```python
from build123d import *

# Parameters (mm, degrees)
SKETCH1_W           = 12.7
SKETCH1_H           = 12.7
BOSS_EXTRUDE1_DEPTH = 6.35
SKETCH2_W           = 1.016
SKETCH2_H           = 3.5052
BOSS_EXTRUDE2_DEPTH = 6.35
FILLET1_R           = 0.635
FILLET2_R           = 0.254


with BuildPart() as part:
    # Sketch1 → Boss-Extrude1 (new body)
    with BuildSketch(Plane(origin=(0, 0, 0), x_dir=(1, 0, 0), z_dir=(0, 1, 0))):
        Rectangle(SKETCH1_W, SKETCH1_H)
    extrude(amount=BOSS_EXTRUDE1_DEPTH)

    # Sketch2 → Boss-Extrude2 (add)
    with BuildSketch(Plane.XY.offset(6.35)):
        with Locations((-2.624666667, 3.175)):
            Rectangle(SKETCH2_W, SKETCH2_H)
        with Locations((2.624666667, 3.175)):
            Rectangle(SKETCH2_W, SKETCH2_H)
    extrude(amount=BOSS_EXTRUDE2_DEPTH)

    # Fillet1
    fillet1_edges = [part.edges().sort_by_distance(p)[0] for p in [
        (-2.624666667, 1.4224, 12.7),
        (-2.624666667, 4.9276, 12.7),
        (2.624666667, 4.9276, 12.7),
        (2.624666667, 1.4224, 12.7),
    ]]
    fillet(fillet1_edges, radius=FILLET1_R)

    # Fillet2
    fillet2_edges = [part.edges().sort_by_distance(p)[0] for p in [
        (6.35, 3.175, 6.35),
        (-6.35, 3.175, 6.35),
        (-6.35, 3.175, -6.35),
        (6.35, 3.175, -6.35),
    ]]
    fillet(fillet2_edges, radius=FILLET2_R)


solid = part.part
```
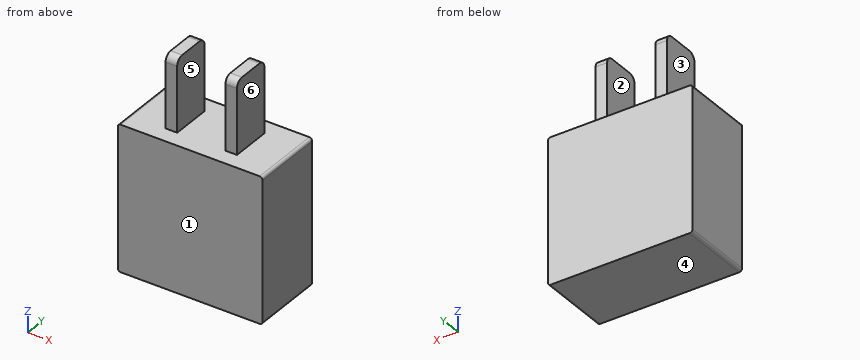
Here's how the part is built. I have some questions about the finished solid (model axes, mm). Face numbers are marked on the shaded views. A direction names the side the tool comes from. Round coordinates to 2 decimals unless told otherwise and drop trailing zeros. Write each loop counter-clockwise with the first axis right and the second up, starting at its lowest first coordinate (ties: lowest second). Pieces come first, ordered by that corner, then holes. Notation, with made-up numbers: M 49,26 L 84,26 A27 cw 84,59 Z; hole C -21,-7 d2. An arc over 180 degrees is marked long. Answer as CSV lines item,"result". Start each with the question number.
1. Suppose I cut it at C-C on x = 5.75. Write out the boundary of the cut face in (y, z).
2. I need wall thicknesses on probe 1 along X at (y, z) = (3, 8.25); probe 2 along Z at (x, y) = (4, 1). Which ranges of each line are inside material? Lowest first, please.
3. Thinking about a two-plate mould opening in X: for the marked faces 1, 2 and 3, which applies, released by +X, released by -X, zero draft, split by the parting line, or undercut?
4. Suppose I cut it at D-D on y = 1.75. Write out the boundary of the cut face in (x, z).
5. I'm going to push flat-ended pins straight in: pin 1 Ø1.8 at (y, z) = (2.5, 9) entering from -X; pin 2 Ø0.8 at (x, z) = (-3, 10) entering from -Y; pin 3 Ø3 at (y, z) = (3.5, 10.5) entering from +X. Where does each tip first touch, or does it pass through?
6. On a 3-axis mill with a long thin cutter (end or side, diameter ignored), from which of +Z, -Z, +X, -X, +Y, -Y can I reach the whole of each face in a straight line? I mean the marked faces 4, 5 and 6. Say none if no direction works.
7. Suppose I cut it at B-B on y = 5.25. Write out the boundary of the cut face in (x, z).
8. Suppose I cut it at A-A on z = 7.75. Write out the boundary of the cut face in (x, y).
Check result:
1,outline,"M 0,-6.35 L 6.35,-6.35 L 6.35,6.35 L 0,6.35 Z"
2,probe 1,"x = -3.13 to -2.12, 2.12 to 3.13"
2,probe 2,"z = -6.35 to 6.35"
3,face 1,"zero draft"
3,face 2,"undercut"
3,face 3,"released by -X"
4,outline,"M -6.35,-6.1 A0.25 ccw -6.1,-6.35 L 6.1,-6.35 A0.25 ccw 6.35,-6.1 L 6.35,6.1 A0.25 ccw 6.1,6.35 L 3.13,6.35 L 3.13,12.62 L 2.12,12.62 L 2.12,6.35 L -2.12,6.35 L -2.12,12.62 L -3.13,12.62 L -3.13,6.35 L -6.1,6.35 A0.25 ccw -6.35,6.1 Z"
5,pin 1,"stops at x = -3.13"
5,pin 2,"stops at y = 1.42"
5,pin 3,"stops at x = 3.13"
6,face 4,"-Z, +X, -X, +Y, -Y"
6,face 5,"+Z, +Y, -Y"
6,face 6,"+Z, +X, +Y, -Y"
7,outline,"M -6.35,-6.1 A0.25 ccw -6.1,-6.35 L 6.1,-6.35 A0.25 ccw 6.35,-6.1 L 6.35,6.1 A0.25 ccw 6.1,6.35 L -6.1,6.35 A0.25 ccw -6.35,6.1 Z"
8,outline,"M -3.13,1.42 L -2.12,1.42 L -2.12,4.93 L -3.13,4.93 Z; M 2.12,1.42 L 3.13,1.42 L 3.13,4.93 L 2.12,4.93 Z"
